Geometry check sheet. Reference: the model listing, model coordinates, mm. Face numbers are marked on the shaded views. A direction names the side the tool comes from. Give positions to 0.01 mm unless a question says otherwise; leave off trailing zeros. Loops run counter-clockwise (first coordinate to the right, second up) from the corner with the lowest first, then second, coordinate; pieces in that order, holes last. Notation, with made-up numbers: (16, 30.25) -> (74, 30.25) arc R28 cw to (74, 56.25) -> close; hole circle Ø7 at (11, 10). An arc over 180 degrees is marked (long way). One line per item, written item: value. Start each with the question number.
(1) Draft check along Y on the marked faces 1, 2 and 3. Enter one of: pulls with the +Y half, pulls with the -Y half, needs draft (parallel to the pull), parting line crosses it, or undercut.
(2) Scan lines: line 1 along X through (y, z) = (20, 39); line 2 along Y through (x, z) = (11.5, 30.5); line 3 along X through (y, z) = (13, 36). Record each from-to range of solid material in increasing order. Write a range as from..to.
(3) Gauge pin test, flat ends, axial feed: pin 1 Ø2 at (x, z) = (2, 36.5) entering from +Y; pin 2 Ø2 at (y, z) = (2.5, 30.5) entering from -X; pin 3 Ø1.3 at (x, z) = (2.5, 20.5) entering from -Y. Record the tip position at first contact, or that the pin passes through.
(4) Tool access check on the marked faces 4, 5, 6 and 7. Record the directions out of +Z, -Z, +X, -X, +Y, -Y that give a thin tool (end or side, any length) a straight path to the whole face; none if there is none.
(5) Sectioned sample at C-C, the plane x = 13.5. Record the cut outline in (y, z).
(6) Sectioned sample at A-A, the plane x = 20. Record the cut outline in (y, z), then the cut area to 3 significant figures.
from build123d import *

# Parameters (mm, degrees)
SKETCH2_R           = 3.492543695
BOSS_EXTRUDE1_DEPTH = 52


with BuildPart() as part:
    # Sketch2 → Boss-Extrude1 (new body)
    with BuildSketch(Plane.XY):
        with BuildLine():
            Line((19.48831917, 27.684671829), (23.749889801, 27.684671829))
            Line((23.749889801, 27.684671829), (29.699681879, 33.624984685))
            ThreePointArc((29.699681879, 33.624984685), (29.917171057, 34.714970099), (28.993139054, 35.332654972))
            Line((28.993139054, 35.332654972), (24.845630957, 35.332654972))
            ThreePointArc((24.845630957, 35.332654972), (24.138524175, 35.625548191), (23.845630957, 36.332654972))
            Line((23.845630957, 36.332654972), (23.845630957, 39))
            ThreePointArc((23.845630957, 39), (24.138524175, 39.707106781), (24.845630957, 40))
            Line((24.845630957, 40), (36, 40))
            ThreePointArc((36, 40), (38.828427125, 38.828427125), (40, 36))
            Line((40, 36), (40, 24.961087436))
            ThreePointArc((40, 24.961087436), (39.707106781, 24.253980655), (39, 23.961087436))
            Line((39, 23.961087436), (36.388269628, 23.961087436))
            ThreePointArc((36.388269628, 23.961087436), (35.681162846, 24.253980655), (35.388269628, 24.961087436))
            Line((35.388269628, 24.961087436), (35.388269628, 29.408620307))
            ThreePointArc((35.388269628, 29.408620307), (34.744223919, 30.343123673), (33.641676542, 30.073901274))
            Line((33.641676542, 30.073901274), (27.684671829, 23.388818206))
            Line((27.684671829, 23.388818206), (27.684671829, 20.51168083))
            Line((27.684671829, 20.51168083), (27.684671829, 16.250110199))
            Line((27.684671829, 16.250110199), (33.624984685, 10.300318121))
            ThreePointArc((33.624984685, 10.300318121), (34.714970099, 10.082828943), (35.332654972, 11.006860946))
            Line((35.332654972, 11.006860946), (35.332654972, 15.154369043))
            ThreePointArc((35.332654972, 15.154369043), (35.625548191, 15.861475825), (36.332654972, 16.154369043))
            Line((36.332654972, 16.154369043), (39, 16.154369043))
            ThreePointArc((39, 16.154369043), (39.707106781, 15.861475825), (40, 15.154369043))
            Line((40, 15.154369043), (40, 4))
            ThreePointArc((40, 4), (38.828427125, 1.171572875), (36, 0))
            Line((36, 0), (24.961087436, 0))
            ThreePointArc((24.961087436, 0), (24.253980655, 0.292893219), (23.961087436, 1))
            Line((23.961087436, 1), (23.961087436, 3.611730372))
            ThreePointArc((23.961087436, 3.611730372), (24.253980655, 4.318837154), (24.961087436, 4.611730372))
            Line((24.961087436, 4.611730372), (29.408620307, 4.611730372))
            ThreePointArc((29.408620307, 4.611730372), (30.343123673, 5.255776081), (30.073901274, 6.358323458))
            Line((30.073901274, 6.358323458), (23.388818206, 12.315328171))
            Line((23.388818206, 12.315328171), (20.51168083, 12.315328171))
            Line((20.51168083, 12.315328171), (16.250110199, 12.315328171))
            Line((16.250110199, 12.315328171), (10.300318121, 6.375015315))
            ThreePointArc((10.300318121, 6.375015315), (10.082828943, 5.285029901), (11.006860946, 4.667345028))
            Line((11.006860946, 4.667345028), (15.154369043, 4.667345028))
            ThreePointArc((15.154369043, 4.667345028), (15.861475825, 4.374451809), (16.154369043, 3.667345028))
            Line((16.154369043, 3.667345028), (16.154369043, 1))
            ThreePointArc((16.154369043, 1), (15.861475825, 0.292893219), (15.154369043, 0))
            Line((15.154369043, 0), (4, 0))
            ThreePointArc((4, 0), (1.171572875, 1.171572875), (0, 4))
            Line((0, 4), (0, 15.038912564))
            ThreePointArc((0, 15.038912564), (0.292893219, 15.746019345), (1, 16.038912564))
            Line((1, 16.038912564), (3.611730372, 16.038912564))
            ThreePointArc((3.611730372, 16.038912564), (4.318837154, 15.746019345), (4.611730372, 15.038912564))
            Line((4.611730372, 15.038912564), (4.611730372, 10.591379693))
            ThreePointArc((4.611730372, 10.591379693), (5.255776081, 9.656876327), (6.358323458, 9.926098726))
            Line((6.358323458, 9.926098726), (12.315328171, 16.611181794))
            Line((12.315328171, 16.611181794), (12.315328171, 19.48831917))
            Line((12.315328171, 19.48831917), (12.315328171, 23.749889801))
            Line((12.315328171, 23.749889801), (6.375015315, 29.699681879))
            ThreePointArc((6.375015315, 29.699681879), (5.285029901, 29.917171057), (4.667345028, 28.993139054))
            Line((4.667345028, 28.993139054), (4.667345028, 24.845630957))
            ThreePointArc((4.667345028, 24.845630957), (4.374451809, 24.138524175), (3.667345028, 23.845630957))
            Line((3.667345028, 23.845630957), (1, 23.845630957))
            ThreePointArc((1, 23.845630957), (0.292893219, 24.138524175), (0, 24.845630957))
            Line((0, 24.845630957), (0, 36))
            ThreePointArc((0, 36), (1.171572875, 38.828427125), (4, 40))
            Line((4, 40), (15.038912564, 40))
            ThreePointArc((15.038912564, 40), (15.746019345, 39.707106781), (16.038912564, 39))
            Line((16.038912564, 39), (16.038912564, 36.388269628))
            ThreePointArc((16.038912564, 36.388269628), (15.746019345, 35.681162846), (15.038912564, 35.388269628))
            Line((15.038912564, 35.388269628), (10.591379693, 35.388269628))
            ThreePointArc((10.591379693, 35.388269628), (9.656876327, 34.744223919), (9.926098726, 33.641676542))
            Line((9.926098726, 33.641676542), (16.611181794, 27.684671829))
            Line((16.611181794, 27.684671829), (19.48831917, 27.684671829))
        make_face()
        with Locations(Location((20, 20, 0), (0, 0, 180))):
            Circle(SKETCH2_R, mode=Mode.SUBTRACT)
    extrude(amount=BOSS_EXTRUDE1_DEPTH)


solid = part.part
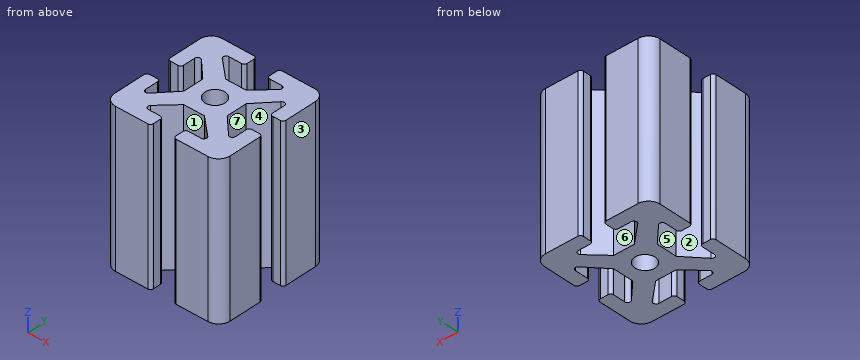
Calculated:
1. face 1: pulls with the -Y half
1. face 2: undercut
1. face 3: needs draft
2. line 1: x = 12.32..16.51, 23.49..27.68
2. line 2: y = 0..4.67, 7.57..15.7, 24.57..32.24, 35.39..40
2. line 3: x = 0..4.61, 9.1..30.93, 35.33..40
3. pin 1: stops at y = 39.87
3. pin 2: stops at x = 0.03
3. pin 3: stops at y = 0.09
4. face 4: +Z, -Z
4. face 5: +Z, -Z, -X
4. face 6: +Z, -Z, +Y
4. face 7: +Z, -Z, +X
5. outline: (0, 0) -> (4.67, 0) -> (4.67, 52) -> (0, 52) -> close; (9.57, 0) -> (30.46, 0) -> (30.46, 52) -> (9.57, 52) -> close; (35.39, 0) -> (40, 0) -> (40, 52) -> (35.39, 52) -> close
6. outline: (12.32, 0) -> (16.51, 0) -> (16.51, 52) -> (12.32, 52) -> close; (23.49, 0) -> (27.68, 0) -> (27.68, 52) -> (23.49, 52) -> close
6. area: 436 mm2
